Here's how the part is built. I have some questions about the finished solid (model axes, mm). Face numbers are marked on the shaded views. A direction names the side the tool comes from. Give positions to 0.01 mm unless a question says otherwise; leave off trailing zeros. Loops run counter-clockwise (first coordinate to the right, second up) from the corner with the lowest first, then second, coordinate; pieces in that order, holes last. Notation, with made-up numbers: M 14,50 L 68,50 A18 ccw 68,67 Z; hole C 44.5,-39.75 d8. An arc over 180 degrees is marked long. Answer as CSV lines item,"result". Start each with the question number.
Item 1: I want a section at B-B on x = 48.5. List the corners of the cut face in (y, z) for me.
Item 2: Will these pins go through, and if not, where does the flat tip stop? P1, Ø1.5, axis at x = 16, z = 4, coming from the -Y side; P2, Ø3, axis at y = 11, z = 5, coming from the +X side; P3, Ø3, axis at x = 89, y = 5, coming from the +Z side.
Item 3: For the marked faces 1 and 2, which set-ups out of +Z, -Z, +X, -X, +Y, -Y let a thin tool reach every point of the face, with its end or its side?
Item 4: If I drill on line 1 along Y through (x, z) = (89, 3.2); line 2 along Y through (x, z) = (90, 2.7); line 3 along X through (y, z) = (6, 1.7), over which ranges is the centre line in solid material (lowest first)? Write a range as from..to.
Item 5: I want a section at C-C on y = 17.25. List the corners of the cut face in (x, z) for me.
Item 6: I want a section at A-A on z = 2.3. List the corners of the cut face in (x, y) for me, plus the area to 3 significant figures.
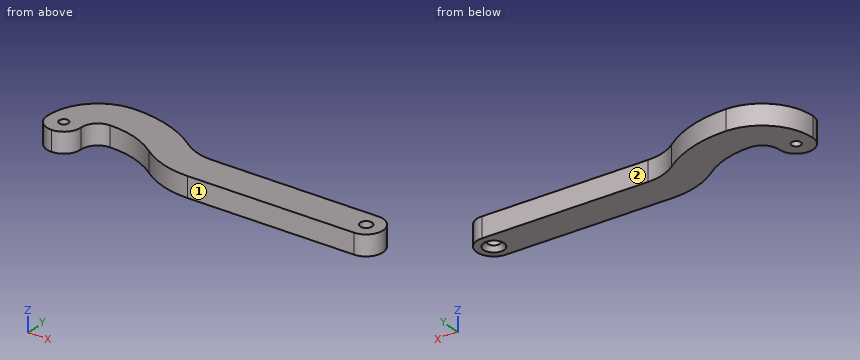
from build123d import *

# Parameters (mm, degrees)
ESQUISSE1_R        = 1.35
ESQUISSE1_R_2      = 1.75
BOSS_EXTRU_1_DEPTH = 6
CHANFREIN1_SIZE    = 1.25


with BuildPart() as part:
    # Esquisse1 → Boss.-Extru.1 (new body)
    with BuildSketch(Plane.XY):
        with BuildLine():
            Line((40, 10), (89, 10))
            ThreePointArc((89, 10), (94, 5), (89, 0))
            Line((89, 0), (40, 0))
            ThreePointArc((40, 0), (32.09430585, 1.282917549), (25, 5))
            ThreePointArc((25, 5), (17.90569415, 8.717082451), (10, 10))
            ThreePointArc((10, 10), (6.464466094, 8.535533906), (5, 5))
            ThreePointArc((5, 5), (3.535533906, 1.464466094), (0, 0))
            ThreePointArc((0, 0), (-3.535533906, 1.464466094), (-5, 5))
            ThreePointArc((-5, 5), (-0.606601718, 15.606601718), (10, 20))
            ThreePointArc((10, 20), (21.067971811, 18.203915432), (31, 13))
            ThreePointArc((31, 13), (35.25658351, 10.769750529), (40, 10))
        make_face()
        with Locations((0, 5)):
            Circle(ESQUISSE1_R, mode=Mode.SUBTRACT)
        with Locations((89, 5)):
            Circle(ESQUISSE1_R_2, mode=Mode.SUBTRACT)
    extrude(amount=BOSS_EXTRU_1_DEPTH)

    # Chanfrein1
    chanfrein1_edges = [part.edges().sort_by_distance(p)[0] for p in [
        (87.25, 5, 0),
    ]]
    chamfer(chanfrein1_edges, length=CHANFREIN1_SIZE)


solid = part.part
Result:
1,outline,"M 0,0 L 10,0 L 10,6 L 0,6 Z"
2,P1,"y = 9.07"
2,P2,"x = 91.18"
2,P3,"through"
3,face 1,"+Z, -Z, +X, -X, -Y"
3,face 2,"+Z, -Z, +X, +Y"
4,line 1,"0..3.25, 6.75..10"
4,line 2,"0.1..3.56, 6.44..9.9"
4,line 3,"-4.97..-0.91, 0.91..5.1, 23.56..87.56, 90.44..93.9"
5,outline,"M 1.34,0 L 23.6,0 L 23.6,6 L 1.34,6 Z"
6,outline,"M -5,5 A5 ccw 5,5 A5 cw 10,10 A25 cw 25,5 A25 ccw 40,0 L 89,0 A5 ccw 89,10 L 40,10 A15 cw 31,13 A35 ccw 10,20 A15 ccw Z; hole C 0,5 d2.7; hole C 89,5 d3.5"
6,area,"1,030 mm^2"
